Geometry check sheet. Reference: the model listing, model coordinates, mm. A direction names the side the tool comes from. Round coordinates to 2 decimals unless told otherwise and drop trailing zeros. Write each loop counter-clockwise with the first axis right and the second up, starting at its lowest first coordinate (ties: lowest second). Pieces come first, ordered by that corner, then holes. Notation, with made-up numbers: (86, -8) -> (126, -8) arc R37 cw to (126, 29) -> close; hole circle Ø8 at (37, 8). An arc over 180 degrees is marked (long way). Use a Markdown table: item, result.
```python
from build123d import *

# Parameters (mm, degrees)
F0_W     = 101.6
F0_H     = 50.8
F1_DEPTH = 3.81
F2_W     = 101.6
F2_H     = 2.54
F3_DEPTH = 2.54
F4_R     = 2.54
F5_DEPTH = 3.81


with BuildPart() as f1:
    # F0 (on Top) → F1 (new body)
    with BuildSketch(Plane.XY):
        with Locations((-1.324669, -1.297615)):
            Rectangle(F0_W, F0_H)
    extrude(amount=-F1_DEPTH)

    # F2 (on face) → F3 (join)
    with BuildSketch(Plane(origin=(0, 0, -3.81), x_dir=(1, 0, 0), z_dir=(0, 0, -1))):
        with Locations((-1.324669, 25.427615)):
            Rectangle(F2_W, F2_H)
        with Locations((-1.324669, -22.832385)):
            Rectangle(F2_W, F2_H)
    extrude(amount=F3_DEPTH)

    # F4 (on face) → F5 (cut)
    with BuildSketch(Plane(origin=(0, 0, -3.81), x_dir=(1, 0, 0), z_dir=(0, 0, -1))):
        with Locations((-39.424669, 19.077615)):
            Circle(F4_R)
        with Locations((-39.424669, -16.482385)):
            Circle(F4_R)
        with Locations((36.775331, 19.077615)):
            Circle(F4_R)
        with Locations((36.775331, -16.482385)):
            Circle(F4_R)
    extrude(amount=-F5_DEPTH, mode=Mode.SUBTRACT)


solid = f1.part
```
(1) Thickness scan on line 1 (Y direction, x = 37.5, z = -1); line 2 (Y direction, x = 22, z = -5.25); line 3 (Z direction, x = 20, y = -5). Record the ranges inside material, lowest first.
A:
| item | result |
|---|---|
| line 1 | y = -26.7 to -21.51, -16.64 to 14.05, 18.92 to 24.1 |
| line 2 | y = -26.7 to -24.16, 21.56 to 24.1 |
| line 3 | z = -3.81 to 0 |
(2) Gauge pin test, flat end, axial feed: pin 1 Ø4 at (x, y) = (-2, 8.5) entering from -Z. Record the tip position at first contact, or that the pin passes through.
A:
| item | result |
|---|---|
| pin 1 | stops at z = -3.81 |
(3) Section check C-C on y = -17.5. Record the cut outline in (x, z).
A:
| item | result |
|---|---|
| outline | (-52.12, -3.81) -> (-41.42, -3.81) -> (-41.42, 0) -> (-52.12, 0) -> close; (-37.43, -3.81) -> (34.78, -3.81) -> (34.78, 0) -> (-37.43, 0) -> close; (38.77, -3.81) -> (49.48, -3.81) -> (49.48, 0) -> (38.77, 0) -> close |
(4) Release check for a two-part mould opening along Y. For faces 3 (the face through (-2, -26.698, -3)), 4 (the face through (-2, 24.102, -3)), 5 (the face through (-2, -1, -3.81)), 6 (the face through (-52.125, -1, -2)) record: +Y half, -Y half, draft (parallel to the pull), parting line (faces both ways), or undercut.
A:
| item | result |
|---|---|
| face 3 | -Y half |
| face 4 | +Y half |
| face 5 | undercut |
| face 6 | draft |
(5) Section check B-B on z = -5. Record the cut outline in (x, y).
A:
| item | result |
|---|---|
| outline | (-52.12, -26.7) -> (49.48, -26.7) -> (49.48, -24.16) -> (-52.12, -24.16) -> close; (-52.12, 21.56) -> (49.48, 21.56) -> (49.48, 24.1) -> (-52.12, 24.1) -> close |
(6) Section check D-D on x = 26. Record the cut outline in (y, z), plus the area to 3 significant figures.
A:
| item | result |
|---|---|
| outline | (-26.7, -6.35) -> (-24.16, -6.35) -> (-24.16, -3.81) -> (21.56, -3.81) -> (21.56, -6.35) -> (24.1, -6.35) -> (24.1, 0) -> (-26.7, 0) -> close |
| area | 206 mm2 |
(7) Access from +Z, -Z, +X, -X, +Y, -Y to the whole of each face (thin tool, end or side, straight path). Record for faces 1 (the face through (-2, 23, -6.35)), 2 (the face through (-2, 21.562, -5)).
A:
| item | result |
|---|---|
| face 1 | -Z, +X, -X, +Y, -Y |
| face 2 | -Z, +X, -X |
(8) Section check A-A on x = -39. Record the cut outline in (y, z).
A:
| item | result |
|---|---|
| outline | (-26.7, -6.35) -> (-24.16, -6.35) -> (-24.16, -3.81) -> (-21.58, -3.81) -> (-21.58, 0) -> (-26.7, 0) -> close; (-16.57, -3.81) -> (13.98, -3.81) -> (13.98, 0) -> (-16.57, 0) -> close; (18.99, -3.81) -> (21.56, -3.81) -> (21.56, -6.35) -> (24.1, -6.35) -> (24.1, 0) -> (18.99, 0) -> close |
